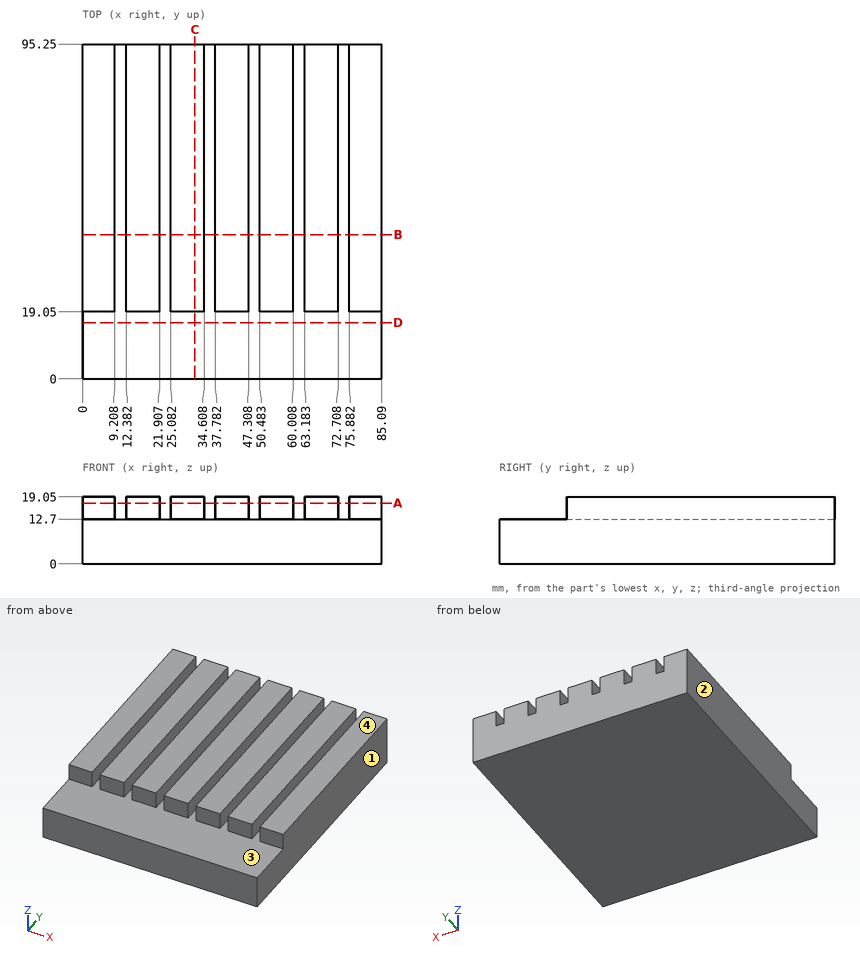
Job drawing, mm, ordinate dimensions from the low corner. One solid piece. Coordinates: 2 decimals unless noted, no trailing zeros. Write each loop counter-clockwise with the first axis right and the second up, starting at its lowest first coordinate (ties: lowest second). Pieces come first, ordered by that corner, then holes. Notation, with made-up numbers: (-1.5, 72.25) -> (47.5, 72.25) arc R25 ccw to (47.5, 107.25) -> close; hole circle Ø11 at (36.25, 16). An arc over 180 degrees is marked (long way). Use CSV: the item, a comma, the result in double quotes. Start each with the question number.
Item 1: Band-saw the part on C-C, the plane x = 32. Write the cut outline in (y, z).
Item 2: Drop flat-ended pins along their axis: P1, Ø8, axis at x = 72.5, z = 2, coming from the -Y side; P2, Ø3, axis at x = 32, z = 15.5, coming from the -Y side. Give the stop position or say it passes through.
Item 3: Two-plate mould, pull along X, no slides. Class the marked faces 1, 2, 3 and 4: +X half, -X half, draft (parallel to the pull), parting line (faces both ways), or undercut.
Item 4: Band-saw the part on D-D, the plane y = 16. Write the cut outline in (x, z).
Item 5: Band-saw the part on B-B, the plane y = 41. Write the cut outline in (x, z).
Item 6: Band-saw the part on A-A, the plane z = 17.25. Write the cut outline in (x, y).
Item 7: Wall check: probe 1 along Z at (x, y) = (74, 53.5); probe 2 along Y at (x, z) = (72, 15). Give the ranges that are in metal, low to high.
Response values:
1,outline,"(0, 0) -> (95.25, 0) -> (95.25, 19.05) -> (19.05, 19.05) -> (19.05, 12.7) -> (0, 12.7) -> close"
2,P1,"stops at y = 0"
2,P2,"stops at y = 19.05"
3,face 1,"+X half"
3,face 2,"-X half"
3,face 3,"undercut"
3,face 4,"draft"
4,outline,"(0, 0) -> (85.09, 0) -> (85.09, 12.7) -> (0, 12.7) -> close"
5,outline,"(0, 0) -> (85.09, 0) -> (85.09, 19.05) -> (75.88, 19.05) -> (75.88, 12.7) -> (72.71, 12.7) -> (72.71, 19.05) -> (63.18, 19.05) -> (63.18, 12.7) -> (60.01, 12.7) -> (60.01, 19.05) -> (50.48, 19.05) -> (50.48, 12.7) -> (47.31, 12.7) -> (47.31, 19.05) -> (37.78, 19.05) -> (37.78, 12.7) -> (34.61, 12.7) -> (34.61, 19.05) -> (25.08, 19.05) -> (25.08, 12.7) -> (21.91, 12.7) -> (21.91, 19.05) -> (12.38, 19.05) -> (12.38, 12.7) -> (9.21, 12.7) -> (9.21, 19.05) -> (0, 19.05) -> close"
6,outline,"(0, 19.05) -> (9.21, 19.05) -> (9.21, 95.25) -> (0, 95.25) -> close; (12.38, 19.05) -> (21.91, 19.05) -> (21.91, 95.25) -> (12.38, 95.25) -> close; (25.08, 19.05) -> (34.61, 19.05) -> (34.61, 95.25) -> (25.08, 95.25) -> close; (37.78, 19.05) -> (47.31, 19.05) -> (47.31, 95.25) -> (37.78, 95.25) -> close; (50.48, 19.05) -> (60.01, 19.05) -> (60.01, 95.25) -> (50.48, 95.25) -> close; (63.18, 19.05) -> (72.71, 19.05) -> (72.71, 95.25) -> (63.18, 95.25) -> close; (75.88, 19.05) -> (85.09, 19.05) -> (85.09, 95.25) -> (75.88, 95.25) -> close"
7,probe 1,"z = 0 to 12.7"
7,probe 2,"y = 19.05 to 95.25"
